Read the model definition and answer for the solid it produces. Units are mm, in the model's axes. Coordinates: 2 decimals unless noted, no trailing zeros. Order: outer loops, then holes, each group sorted by start corner. A loop starts at its lowest first (then second) coordinate and runs counter-clockwise, first axis right, second up.
```python
from build123d import *

# Parameters (mm, degrees)
F0_R     = 1.7272
F0_W     = 24
F0_H     = 12.254687
F1_DEPTH = 3.2512


with BuildPart() as f1:
    # F0 (on Top) → F1 (new body)
    with BuildSketch(Plane.XY):
        Polygon((94.31227, 0), (0, 0), (0, -59.449995), (94.31227, -59.449995), (94.31227, -18.612498), align=None)
        with Locations((3.96875, -55.481245)):
            Circle(F0_R, mode=Mode.SUBTRACT)
        with Locations((3.96875, -39.606245)):
            Circle(F0_R, mode=Mode.SUBTRACT)
        with Locations((11.90625, -33.256245)):
            Circle(F0_R, mode=Mode.SUBTRACT)
        with Locations((34.733674, -41.71249)):
            Circle(F0_R, mode=Mode.SUBTRACT)
        with Locations((42.671175, -43.033084)):
            Circle(F0_R, mode=Mode.SUBTRACT)
        with Locations((27.968753, -33.256245)):
            Circle(F0_R, mode=Mode.SUBTRACT)
        with Locations((58.546175, -43.033084)):
            Circle(F0_R, mode=Mode.SUBTRACT)
        with Locations((66.343517, -33.256245)):
            Circle(F0_R, mode=Mode.SUBTRACT)
        with Locations((75.993511, -41.71249)):
            Circle(F0_R, mode=Mode.SUBTRACT)
        with Locations((82.40602, -33.256245)):
            Circle(F0_R, mode=Mode.SUBTRACT)
        with Locations((19.9375, -18.612497)):
            Rectangle(F0_W, F0_H, mode=Mode.SUBTRACT)
        with Locations((3.96875, -3.96875)):
            Circle(F0_R, mode=Mode.SUBTRACT)
        with Locations((11.90625, -3.96875)):
            Circle(F0_R, mode=Mode.SUBTRACT)
        with Locations((19.84375, -3.96875)):
            Circle(F0_R, mode=Mode.SUBTRACT)
        with Locations((27.968753, -3.96875)):
            Circle(F0_R, mode=Mode.SUBTRACT)
        Polygon((86.37477, -12.485154), (86.37477, -18.612498), (86.37477, -24.739841), (62.37477, -24.739841), (62.37477, -12.485154), align=None, mode=Mode.SUBTRACT)
        with Locations((66.343517, -3.96875)):
            Circle(F0_R, mode=Mode.SUBTRACT)
        with Locations((74.46852, -3.96875)):
            Circle(F0_R, mode=Mode.SUBTRACT)
        with Locations((82.40602, -3.96875)):
            Circle(F0_R, mode=Mode.SUBTRACT)
        with Locations((90.34352, -3.96875)):
            Circle(F0_R, mode=Mode.SUBTRACT)
    extrude(amount=F1_DEPTH)


solid = f1.part
```
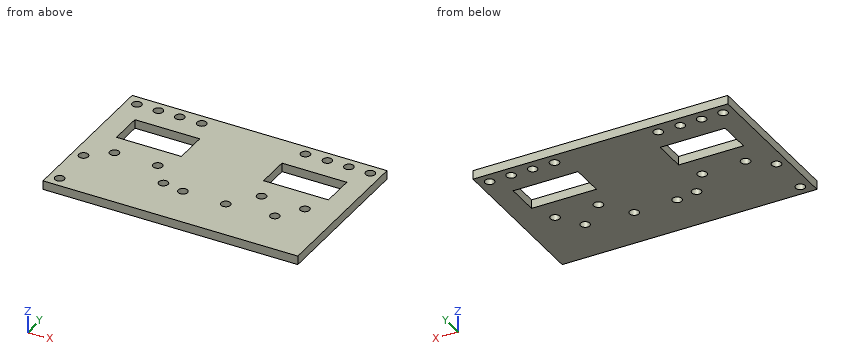
1) A cutting plane is placed at A-A, the plane x = 70. Determine the outline of the cut face in (y, z), and give its area (3 significant figures).
A:
outline: (-59.45, 0) - (-24.74, 0) - (-24.74, 3.25) - (-59.45, 3.25) - close; (-12.49, 0) - (0, 0) - (0, 3.25) - (-12.49, 3.25) - close
area: 153 mm2
2) A cutting plane is placed at C-C, the plane x = 28. Determine the outline of the cut face in (y, z), and give its area (3 significant figures).
A:
outline: (-59.45, 0) - (-34.98, 0) - (-34.98, 3.25) - (-59.45, 3.25) - close; (-31.53, 0) - (-24.74, 0) - (-24.74, 3.25) - (-31.53, 3.25) - close; (-12.49, 0) - (-5.7, 0) - (-5.7, 3.25) - (-12.49, 3.25) - close; (-2.24, 0) - (0, 0) - (0, 3.25) - (-2.24, 3.25) - close
area: 131 mm2
3) Straight lines are drawn through the part: line 1 (X direction, y = -17.5, z = 1.45); line 2 (Y direction, x = 28, z = 1.5); line 3 (Y direction, x = 34.5, z = 2.6). For each, find the intervals that lie inside material, in ascending order.
A:
line 1: x = 0 to 7.94, 31.94 to 62.37, 86.37 to 94.31
line 2: y = -59.45 to -34.98, -31.53 to -24.74, -12.49 to -5.7, -2.24 to 0
line 3: y = -59.45 to -43.42, -40 to 0
4) A cutting plane is placed at D-D, the plane z = 1.5. State how many separate pieces and enclosed holes the cut face has, and give its area (3 significant figures).
A:
separate pieces: 1
enclosed holes: 20
area: 4,850 mm2
5) A cutting plane is placed at B-B, the plane y = -20.5. Determine the outline of the cut face in (x, z).
A:
outline: (0, 0) - (7.94, 0) - (7.94, 3.25) - (0, 3.25) - close; (31.94, 0) - (62.37, 0) - (62.37, 3.25) - (31.94, 3.25) - close; (86.37, 0) - (94.31, 0) - (94.31, 3.25) - (86.37, 3.25) - close
